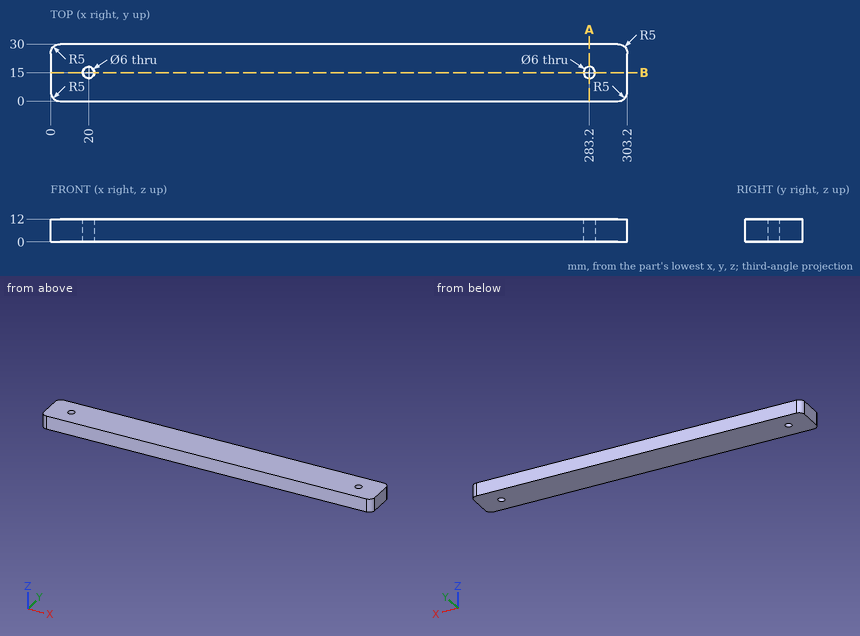
Can you work these out from the drawing? Everything is in mm from the part's minimum corner. Coordinates: 2 decimals unless noted, no trailing zeros. Loops run counter-clockwise (first coordinate to the right, second up) from the corner with the lowest first, then second, coordinate; pieces in that order, holes last.
1) Imagine slicing it at B-B on y = 15. List the corners of the cut face in (x, z) for me, plus the area to 3 significant figures.
2) Imagine slicing it at A-A on x = 283.2. List the corners of the cut face in (y, z) for me.
3) For pin 1 (2 mm diameter, centred on x = 97.5, z = 2.5, fed in from -Y), with a flat end and sliding along its axis, tell me the tip position at first contact or that it passes through.
4) I need wall thicknesses on probe 1 along Y at (x, z) = (283.2, 7.5); probe 2 along X at (y, z) = (14.5, 11.75); probe 3 along X at (y, z) = (13.5, 9.25). Which ranges of each line are inside material? Lowest first, please.
Completed:
1. outline: (0, 0) - (17, 0) - (17, 12) - (0, 12) - close; (23, 0) - (280.2, 0) - (280.2, 12) - (23, 12) - close; (286.2, 0) - (303.2, 0) - (303.2, 12) - (286.2, 12) - close
1. area: 3,490 mm2
2. outline: (0, 0) - (12, 0) - (12, 12) - (0, 12) - close; (18, 0) - (30, 0) - (30, 12) - (18, 12) - close
3. pin 1: stops at y = 0
4. probe 1: y = 0 to 12, 18 to 30
4. probe 2: x = 0 to 17.04, 22.96 to 280.24, 286.16 to 303.2
4. probe 3: x = 0 to 17.4, 22.6 to 280.6, 285.8 to 303.2
